The model under review builds one solid part; all positions refer to its coordinate system, in mm. A direction names the side the tool comes from. Give positions to 0.01 mm unless a question says otherwise; leave off trailing zeros. Write each loop counter-clockwise with the first axis right and the second up, starting at its lowest first coordinate (ties: lowest second). Pieces come first, ordered by that corner, then holes. Notation, with made-up numbers: (51, 3.5) - (109, 3.5) arc R24 ccw to (109, 21.5) - close; hole circle Ø10 at (-20.5, 63). An arc over 180 degrees is marked (long way). Write item = value, one per line.
```python
from build123d import *

# Parameters (mm, degrees)
SKETCH1_W                = 70
SKETCH1_H                = 110
BOSS_EXTRUDE1_DEPTH      = 8
BOSS_EXTRUDE2_DEPTH      = 18
SKETCH3_R                = 1.3
CUT_EXTRUDE1_DEPTH       = 133.951118837
CUT_EXTRUDE3_START       = -6
SKETCH4_R                = 2.45
CUT_EXTRUDE3_DEPTH       = 127.951118837
CHAMFER2_SIZE            = 6
CHAMFER7_SIZE            = 4
CHAMFER6_SIZE            = 2.5
SKETCH6_W                = 10
SKETCH6_H                = 50
BOSS_EXTRUDE4_DEPTH      = 30.3
BOSS_EXTRUDE5_START      = 5
SKETCH7_W                = 16.5
SKETCH7_H                = 50
SKETCH7_R                = 1.3
BOSS_EXTRUDE5_DEPTH      = 5
SKETCH8_W                = 6.5
SKETCH8_H                = 30.3
BOSS_EXTRUDE6_DEPTH      = 5
BOSS_EXTRUDE7_DEPTH      = 4
BOSS_EXTRUDE7_DEPTH_BACK = 4


with BuildPart() as part:
    # Sketch1 → Boss-Extrude1 (new body)
    with BuildSketch(Plane(origin=(0, 0, 0), x_dir=(1, 0, 0), z_dir=(0, 1, 0))):
        with Locations((35, 55)):
            Rectangle(SKETCH1_W, SKETCH1_H)
    extrude(amount=BOSS_EXTRUDE1_DEPTH)

    # Sketch2 → Boss-Extrude2 (add)
    with BuildSketch(Plane(origin=(0, 8, 0), x_dir=(1, 0, 0), z_dir=(0, 1, 0))):
        Polygon((70, 67.35), (40, 67.35), (40, 42.65), (70, 42.65), (70, 30), (23, 30), (23, 80), (70, 80), align=None)
    extrude(amount=BOSS_EXTRUDE2_DEPTH)

    # Sketch3 → Cut-Extrude1 (cut, through all)
    with BuildSketch(Plane(origin=(0, 26, 0), x_dir=(1, 0, 0), z_dir=(0, 1, 0))):
        with Locations(Location((60.5, 70, 0), (0, 0, 270))):
            Circle(SKETCH3_R)
        with Locations(Location((37.2, 63.5, 0), (0, 0, 270))):
            Circle(SKETCH3_R)
    cut_extrude1 = extrude(amount=-CUT_EXTRUDE1_DEPTH, mode=Mode.SUBTRACT)

    # Sketch4 → Cut-Extrude3 (cut, through all)
    with BuildSketch(Plane(origin=(0, 26, 0), x_dir=(1, 0, 0), z_dir=(0, 1, 0)).offset(CUT_EXTRUDE3_START)):
        with Locations(Location((37.2, 63.5, 0), (0, 0, 270))):
            Circle(SKETCH4_R)
        with Locations(Location((60.5, 70, 0), (0, 0, 270))):
            Circle(SKETCH4_R)
    cut_extrude3 = extrude(amount=-CUT_EXTRUDE3_DEPTH, mode=Mode.SUBTRACT)

    # Mirror3: Cut-Extrude1, Cut-Extrude3 across plane
    add(cut_extrude1.mirror(Plane.XY.offset(-55)), mode=Mode.SUBTRACT)
    add(cut_extrude3.mirror(Plane.XY.offset(-55)), mode=Mode.SUBTRACT)

    # Chamfer2
    chamfer2_edges = [part.edges().sort_by_distance(p)[0] for p in [
        (70, 17, -67.35),
        (70, 17, -42.65),
    ]]
    chamfer(chamfer2_edges, length=CHAMFER2_SIZE)

    # Chamfer7
    chamfer7_edges = [part.edges().sort_by_distance(p)[0] for p in [
        (70, 17, -80),
        (70, 17, -30),
    ]]
    chamfer(chamfer7_edges, length=CHAMFER7_SIZE)

    # Chamfer6
    chamfer6_edges = [part.edges().sort_by_distance(p)[0] for p in [
        (44.5, 8, -80),
        (68, 8, -78),
        (68, 8, -32),
        (23, 8, -55),
        (44.5, 8, -30),
    ]]
    chamfer(chamfer6_edges, length=CHAMFER6_SIZE)

    # Sketch6 → Boss-Extrude4 (add)
    with BuildSketch(Plane(origin=(0, 26, 0), x_dir=(1, 0, 0), z_dir=(0, 1, 0))):
        with Locations((28, 55)):
            Rectangle(SKETCH6_W, SKETCH6_H)
    extrude(amount=BOSS_EXTRUDE4_DEPTH)

    # Sketch7 → Boss-Extrude5 (add)
    with BuildSketch(Plane(origin=(0, 56.3, 0), x_dir=(1, 0, 0), z_dir=(0, 1, 0)).offset(BOSS_EXTRUDE5_START)):
        with Locations((31.25, 55)):
            Rectangle(SKETCH7_W, SKETCH7_H)
        with Locations(Location((37.2, 63.5, 0), (0, 0, 270))):
            Circle(SKETCH7_R, mode=Mode.SUBTRACT)
        with Locations(Location((37.2, 46.5, 0), (0, 0, 270))):
            Circle(SKETCH7_R, mode=Mode.SUBTRACT)
    extrude(amount=-BOSS_EXTRUDE5_DEPTH)

    # Sketch8 → Boss-Extrude6 (add)
    with BuildSketch(Plane.XY.offset(-30)):
        with Locations((36.25, 41.15)):
            Rectangle(SKETCH8_W, SKETCH8_H)
    boss_extrude6 = extrude(amount=-BOSS_EXTRUDE6_DEPTH)

    # Mirror4: Boss-Extrude6 across plane
    add(boss_extrude6.mirror(Plane.XY.offset(-55)))

    # Sketch9 → Boss-Extrude7 (add, two sides: drawn at the far end of the back side and taken through both)
    with BuildSketch(Plane.XY.offset(-55).offset(-BOSS_EXTRUDE7_DEPTH_BACK)):
        Polygon((0, 8), (23, 8), (23, 61.3), align=None)
    extrude(amount=BOSS_EXTRUDE7_DEPTH + BOSS_EXTRUDE7_DEPTH_BACK)


solid = part.part
```
1. Take a section at D-D on y = 45. Give the boundary of the cut face in (x, z), and give its area (3 significant figures).
Findings below:
outline = (15.97, -59) - (23, -59) - (23, -80) - (39.5, -80) - (39.5, -75) - (33, -75) - (33, -35) - (39.5, -35) - (39.5, -30) - (23, -30) - (23, -51) - (15.97, -51) - close
area = 621 mm²
2. Take a section at C-C on y = 17.5. Give the boundary of the cut face in (x, z), and give its area (3 significant figures).
Findings below:
outline = (4.1, -59) - (23, -59) - (23, -80) - (66, -80) - (70, -76) - (70, -73.35) - (64, -67.35) - (40, -67.35) - (40, -42.65) - (64, -42.65) - (70, -36.65) - (70, -34) - (66, -30) - (23, -30) - (23, -51) - (4.1, -51) - close; hole circle Ø4.9 at (37.2, -63.5); hole circle Ø4.9 at (37.2, -46.5); hole circle Ø4.9 at (60.5, -70); hole circle Ø4.9 at (60.5, -40)
area = 1,630 mm²
3. Insertion check: P1, Ø10.5, axis at y = 34.5, z = -71.5, coming from the -X side; P2, Ø18.5, axis at x = 13, y = 40.5, coming from the -Z side; P3, Ø9, axis at x = 48.5, y = 19.5, coming from the -Z side; P4, Ø2.5, axis at x = 37.2, z = -46.5, coming from the +Y side. Each pin has a flat end and moves straight along its axis. Give the tip position at first contact, or say it passes through.
Findings below:
P1 = 23
P2 = -59
P3 = -80
P4 = through
4. Draft analysis for pull direction X (two halves, no side actions). For faces 1 (the flat face through (0, 4, -54)), 2 (the cylindrical face through (36.262, 10.14, -48.763)), 3 (the flat face through (36, 20, -62)), 4 (the flat face through (39, 26, -55)), state which applies: +X half, -X half, draft (parallel to the pull), parting line (faces both ways), or undercut.
Findings below:
face_1 = -X half
face_2 = undercut
face_3 = undercut
face_4 = draft
5. Machinability: for faces 5 (the flat face through (66.96, 16.87, -39.69)), 6 (the flat face through (33, 41, -55)), 7 (the flat face through (39, 31, -30)), 8 (the flat face through (16, 23, -59)), which of the approach directions +Z, -Z, +X, -X, +Y, -Y give a long, thin tool a straight path to every point of the face, cutting with its end or side? Answer none if there is none.
Findings below:
face_5 = +X, +Y
face_6 = +X
face_7 = +Z, +X, -X, +Y
face_8 = -Z, -X, +Y
6. For line 1 (Y direction, x = 27, z = -85); line 2 (Y direction, x = 53, z = -35.5); line 3 (Z direction, x = 12, y = 29.5), list the stretches that pass through material, from the lowest coordinate up. Write a range as from..to.
Findings below:
line_1 = 0..8
line_2 = 0..26
line_3 = -59..-51
7. Take a section at B-B on x = 27. Give the boundary of the cut face in (y, z), and give its area (3 significant figures).
Findings below:
outline = (0, -110) - (8, -110) - (8, -82.5) - (10.5, -80) - (61.3, -80) - (61.3, -30) - (10.5, -30) - (8, -27.5) - (8, 0) - (0, 0) - close
area = 3,550 mm²
8. Take a section at A-A on z = -46.5. Give the boundary of the cut face in (x, y), and give its area (3 significant figures).
Findings below:
outline = (0, 0) - (34.75, 0) - (34.75, 20) - (35.9, 20) - (35.9, 26) - (33, 26) - (33, 56.3) - (35.9, 56.3) - (35.9, 61.3) - (23, 61.3) - (23, 10.5) - (20.5, 8) - (0, 8) - close; (38.5, 20) - (39.65, 20) - (39.65, 0) - (70, 0) - (70, 8) - (40, 8) - (40, 26) - (38.5, 26) - close; (38.5, 56.3) - (39.5, 56.3) - (39.5, 61.3) - (38.5, 61.3) - close
area = 1,130 mm²
